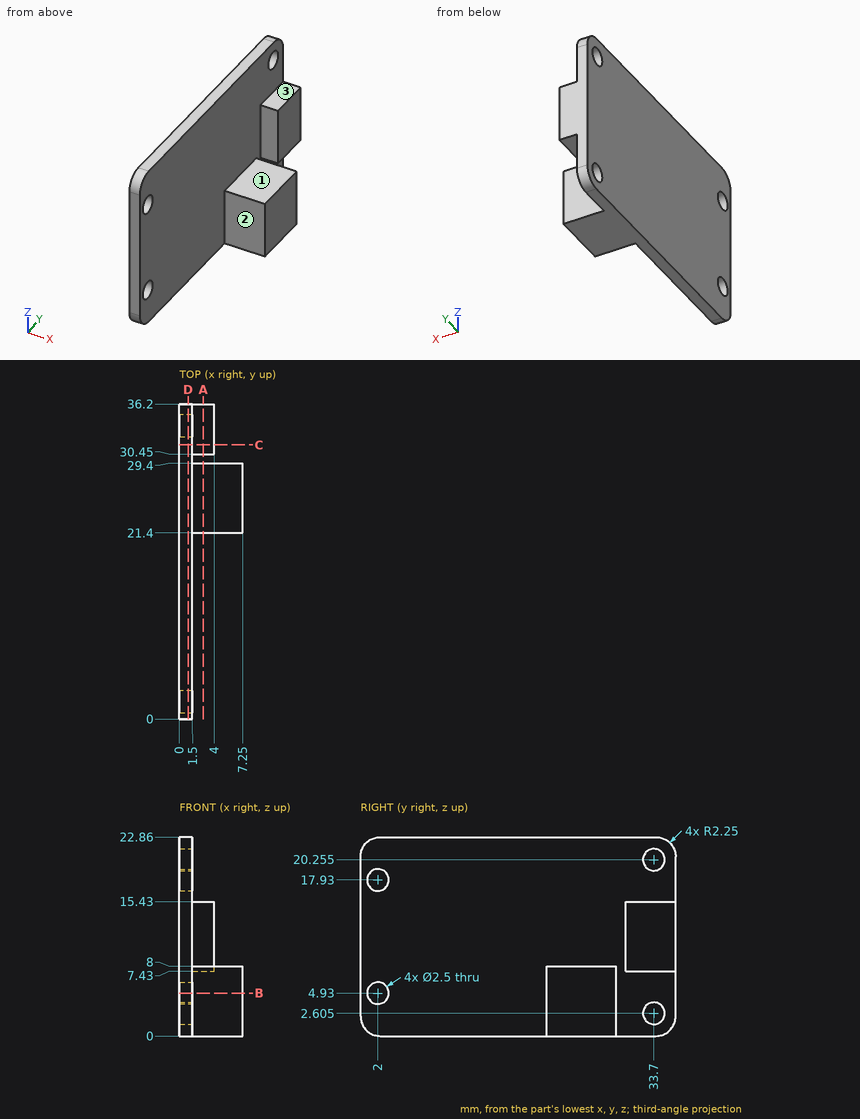
Answer from the drawing. Dimensions are ordinates in mm from the lowest x, y and z of the part. A direction names the side the tool comes from. Coordinates: 2 decimals unless noted, no trailing zeros. Write each loop counter-clockwise with the first axis right and the second up, starting at its lowest first coordinate (ties: lowest second). Pieces come first, ordered by that corner, then holes. Notation, with made-up numbers: (15.5, 31) - (52.5, 31) arc R18 ccw to (52.5, 61) - close; hole circle Ø11 at (78, 60). An arc over 180 degrees is marked (long way). One line per question, with ' | ' between items.
Q1. Consider L1, parallel to Z at x = 0.65, y = 33.7 (3 decimals); L2, parallel to Z at x = 1.1, y = 2; L3, parallel to Y at x = 6, z = 3.5. Determine where each line is inside the solid, lowest interval first. Write a range as [from, to].
Result set:
L1: [0, 1.355], [3.855, 19.005], [21.505, 22.86] | L2: [0.01, 3.68], [6.18, 16.68], [19.18, 22.85] | L3: [21.4, 29.4]
Q2. Find section A-A, the plane x = 2.75. Write down the section's boundary in (y, z), plus the area to 3 significant figures.
Result set:
outline: (21.4, 0) - (29.4, 0) - (29.4, 8) - (21.4, 8) - close; (30.45, 7.43) - (36.2, 7.43) - (36.2, 15.43) - (30.45, 15.43) - close | area: 110 mm^2
Q3. Find section D-D, the plane x = 1. Write down the section's boundary in (y, z) (3 decimals).
Result set:
outline: (0, 2.25) arc R2.25 ccw to (2.25, 0) - (33.95, 0) arc R2.25 ccw to (36.2, 2.25) - (36.2, 20.61) arc R2.25 ccw to (33.95, 22.86) - (2.25, 22.86) arc R2.25 ccw to (0, 20.61) - close; hole circle Ø2.5 at (2, 4.93); hole circle Ø2.5 at (2, 17.93); hole circle Ø2.5 at (33.7, 2.605); hole circle Ø2.5 at (33.7, 20.255)
Q4. Find section B-B, the plane z = 4.93. Write down the section's boundary in (x, y), plus the area to 4 significant figures.
Result set:
outline: (0, 0) - (1.5, 0) - (1.5, 0.75) - (0, 0.75) - close; (0, 3.25) - (1.5, 3.25) - (1.5, 21.4) - (7.25, 21.4) - (7.25, 29.4) - (1.5, 29.4) - (1.5, 36.2) - (0, 36.2) - close | area: 96.55 mm^2
Q5. For the marked faces 1, 2 and 3, determine the directions among +Z, -Z, +X, -X, +Y, -Y from which every point of the face is accessible in a straight line to the end or side of a thin tool.
Result set:
face 1: +Z, +X, -Y | face 2: +Z, -Z, +X, -Y | face 3: +Z, +X, +Y, -Y
Q6. Each of these flat-tipped pins is pushed along its axis until it touches: P1, Ø3, axis at x = 5.5, z = 4, coming from the +Y side; P2, Ø0.8, axis at x = 3, y = 33.5, coming from the -Z side; P3, Ø0.8, axis at x = 2.5, y = 33.5, coming from the +Z side. Where does it stop, or does it pass through?
Result set:
P1: y = 29.4 | P2: z = 7.43 | P3: z = 15.43
Q7. Find section C-C, the plane y = 31.5. Write down the section's boundary in (x, z), plus the area to 3 significant figures.
Result set:
outline: (0, 0) - (1.5, 0) - (1.5, 7.43) - (4, 7.43) - (4, 15.43) - (1.5, 15.43) - (1.5, 22.86) - (0, 22.86) - close | area: 54.3 mm^2
